Here's the drawing with two shaded views (mm, measured from the low corner). I have some questions. A direction names the side the tool comes from. Round coordinates to 2 decimals unless told otherwise and drop trailing zeros. Loops run counter-clockwise (first coordinate to the right, second up) from the corner with the lowest first, then second, coordinate; pieces in that order, holes last.
(1) Will these pins go through, and if not, where does the flat tip stop? pin 1 Ø10 at (y, z) = (49.5, 6.5) entering from +X; pin 2 Ø6 at (x, z) = (68.5, 8.5) entering from +Y.
(2) Which directions (+Z, -Z, +X, -X, +Y, -Y) give clear straight access to the entire face, cutting with the end or side of a thin tool? Please do the marked faces 1 and 2.
(3) I want a section at A-A on z = 3.75. Write out the boundary of the cut face in (x, y), plus the area to 3 significant figures.
(4) I want a section at B-B on x = 79. Write out the boundary of the cut face in (y, z), plus the area to 3 significant figures.
(5) If I drill on line 1 along Y through (x, z) = (51, 14.5); line 2 along X through (y, z) = (50, 13.75), over which ranges is the centre line in solid material (lowest first)?
(6) I want a section at C-C on y = 49. Write out the boundary of the cut face in (x, z), plus the area to 3 significant figures.
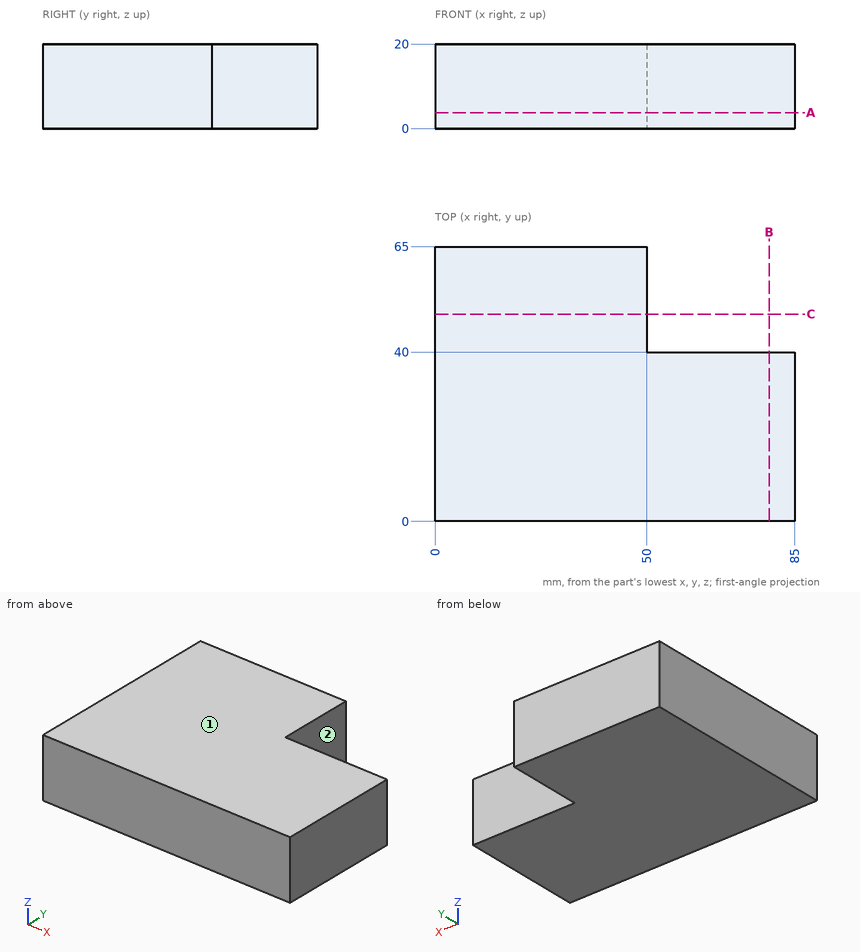
Filled sheet:
1. pin 1: stops at x = 50
1. pin 2: stops at y = 40
2. face 1: +Z, +X, -X, +Y, -Y
2. face 2: +Z, -Z, +X, +Y
3. outline: (0, 0) - (85, 0) - (85, 40) - (50, 40) - (50, 65) - (0, 65) - close
3. area: 4,650 mm2
4. outline: (0, 0) - (40, 0) - (40, 20) - (0, 20) - close
4. area: 800 mm2
5. line 1: y = 0 to 40
5. line 2: x = 0 to 50
6. outline: (0, 0) - (50, 0) - (50, 20) - (0, 20) - close
6. area: 1,000 mm2
